```python
from build123d import *

# Parameters (mm, degrees)
F0_W     = 50.8
F0_H     = 13.97
F1_DEPTH = 19.05
F3_DEPTH = 19.05
F5_DEPTH = 25.4
F6_R     = 3.5000041341
F7_DEPTH = 25.4
F9_DEPTH = 11.43


with BuildPart() as f1:
    # F0 (on Front) → F1 (new body)
    with BuildSketch(Plane.XZ):
        with Locations((0, -6.985)):
            Rectangle(F0_W, F0_H)
    extrude(amount=-F1_DEPTH)

    # F2 (on face) → F3 (cut)
    with BuildSketch(Plane.XZ):
        with BuildLine():
            ThreePointArc((-10.668, 0), (0, -10.668), (10.668, 0))
            Line((10.668, 0), (-10.668, 0))
        make_face()
    extrude(amount=-F3_DEPTH, mode=Mode.SUBTRACT)

    # F4 (on face) → F5 (cut)
    with BuildSketch(Plane.XZ):
        Polygon((-25.4, -3.81), (-25.4, -13.97), (-10.16, -13.97), align=None)
        Polygon((25.4, -13.97), (25.4, -3.81), (10.16, -13.97), align=None)
    extrude(amount=-F5_DEPTH, mode=Mode.SUBTRACT)

    # F6 (on face) → F7 (cut)
    with BuildSketch(Plane.XY):
        with Locations((-17.4625, 9.525)):
            Circle(F6_R)
        with Locations((17.4625, 9.525)):
            Circle(F6_R)
    extrude(amount=-F7_DEPTH, mode=Mode.SUBTRACT)

    # F8 (on face) → F9 (cut)
    with BuildSketch(Plane(origin=(0, 0, -13.97), x_dir=(1, 0, 0), z_dir=(0, 0, -1))):
        Polygon((-14.2547823489, -3.9263508054), (-20.7072136039, -3.9477104287), (-23.9149312549, -9.5463596233), (-20.6702176511, -15.1236491946), (-14.2177863961, -15.1022895713), (-11.0100687451, -9.5036403767), align=None)
        Polygon((23.9149312549, -9.5463596233), (20.7072136039, -3.9477104287), (14.2547823489, -3.9263508054), (11.0100687451, -9.5036403767), (14.2177863961, -15.1022895713), (20.6702176511, -15.1236491946), align=None)
    extrude(amount=-F9_DEPTH, mode=Mode.SUBTRACT)


solid = f1.part
```
The model under review builds one solid part; all positions refer to its coordinate system, in mm. A direction names the side the tool comes from. Coordinates: 2 decimals unless noted, no trailing zeros. Write each loop counter-clockwise with the first axis right and the second up, starting at its lowest first coordinate (ties: lowest second). Pieces come first, ordered by that corner, then holes. Notation, with made-up numbers: (53.25, 16) - (95.25, 16) arc R18 cw to (95.25, 28) - close; hole circle Ø3 at (-38.5, 14.5). An arc over 180 degrees is marked (long way). Answer in a Markdown table with one row per item. Add a question column.
Q1. Consider section B-B on y = 7.5. Give the boundary of the cut face in (x, z).
Q2. To check wall thickness, follow line 1 along X through (y, z) = (12.25, -3.25); line 2 along X through (y, z) = (6.5, -3.5); line 3 along Z through (x, y) = (0.5, 10). State the ranges of each line that lie inside material, in increasing order. Write a range as from..to.
Q3. Draft analysis for pull direction Y (two halves, no side actions). For faces 3 (the face through (-17.673, 3.042, -8.961)), 4 (the face through (-22.29, 6.71, -4.28)), 5 (the face through (0, 19.05, -12)), state which applies: +Y half, -Y half, draft (parallel to the pull), parting line (faces both ways), or undercut.
Q4. Consider section C-C on x = 20. Give the boundary of the cut face in (y, z).
Q5. Consider section A-A on z = -8.75. Give the boundary of the cut face in (x, y).
Q6. Clearance check with flat-ended pins moving along their axes: pin 1 (3 mm diameter, centred on y = 15.5, z = -8.5, fed in from +X) (3 decimals); pin 2 (5.5 mm diameter, centred on x = -18, y = 8.5, fed in from -Z); pin 3 (8 mm diameter, centred on x = 0.5, y = 2, fed in from +Z). State where each tip first meets the part, or that it passes through.
Q7. For faces 1 (the face through (12.655, 6.676, -8.048)), 2 (the face through (-25.4, 9, -2)), list the 3-axis set-ups (+Z, -Z, +X, -X, +Y, -Y) from which the entire face can be reached by the end or side of a thin tool; tool diameter is ignored.
Q8. Consider section D-D on y = 16.25. Give the boundary of the cut face in (x, z), then the cut area to 3 significant figures.
Answers below:
| question | item | result |
|---|---|---|
| 1 | outline | (-25.4, -3.81) - (-22.74, -5.58) - (-22.74, -2.54) - (-20.32, -2.54) - (-20.32, 0) - (-25.4, 0) - close; (-14.61, -2.54) - (-12.18, -2.54) - (-12.18, -12.63) - (-10.16, -13.97) - (10.16, -13.97) - (12.18, -12.63) - (12.18, -2.54) - (14.61, -2.54) - (14.61, 0) - (10.67, 0) arc R10.67 cw to (-10.67, 0) - (-14.61, 0) - close; (20.32, -2.54) - (22.74, -2.54) - (22.74, -5.58) - (25.4, -3.81) - (25.4, 0) - (20.32, 0) - close |
| 2 | line 1 | -25.4..-22.34, -12.58..-10.16, 10.16..12.58, 22.34..25.4 |
| 2 | line 2 | -25.4..-22.17, -12.76..-10.08, 10.08..12.76, 22.17..25.4 |
| 2 | line 3 | -13.97..-10.66 |
| 3 | face 3 | draft |
| 3 | face 4 | undercut |
| 3 | face 5 | +Y half |
| 4 | outline | (0, -7.41) - (3.95, -7.41) - (3.95, -2.54) - (7.11, -2.54) - (7.11, 0) - (0, 0) - close; (11.94, -2.54) - (15.12, -2.54) - (15.12, -7.41) - (19.05, -7.41) - (19.05, 0) - (11.94, 0) - close |
| 5 | outline | (-17.99, 0) - (-6.1, 0) - (-6.1, 19.05) - (-17.99, 19.05) - (-17.99, 15.11) - (-14.22, 15.1) - (-11.01, 9.5) - (-14.25, 3.93) - (-17.99, 3.94) - close; (6.1, 0) - (17.99, 0) - (17.99, 3.94) - (14.25, 3.93) - (11.01, 9.5) - (14.22, 15.1) - (17.99, 15.11) - (17.99, 19.05) - (6.1, 19.05) - close |
| 6 | pin 1 | x = 20.615 |
| 6 | pin 2 | z = -2.54 |
| 6 | pin 3 | z = -9.67 |
| 7 | face 1 | -Z |
| 7 | face 2 | +Z, -Z, -X, +Y, -Y |
| 8 | outline | (-25.4, -3.81) - (-10.16, -13.97) - (10.16, -13.97) - (25.4, -3.81) - (25.4, 0) - (10.67, 0) arc R10.67 cw to (-10.67, 0) - (-25.4, 0) - close |
| 8 | area | 376 mm² |
